from build123d import *

# Parameters (mm, degrees)
EXTRUDE_1_DEPTH     = 14.5
SKETCH_3_W          = 7.5
SKETCH_3_H          = 12.5
CUT_EXTRUDE_1_DEPTH = 14.5
SKETCH_4_W          = 6.236601739
SKETCH_4_H          = 12.5
CUT_EXTRUDE_2_DEPTH = 14.5


with BuildPart() as part:
    # 草图2 → 凸台-拉伸1 (new body)
    with BuildSketch(Plane.XY):
        Polygon((-37.803253111, 45.788749387), (-30.303253111, 45.788749387), (-30.303253111, 46.246753013), (-30.303253111, 51.227331274), (-45.303253111, 51.227331274), (-45.303253111, 45.788749387), align=None)
        with BuildLine():
            Line((-36.53985485, 45.788749387), (-37.803253111, 45.788749387))
            Line((-37.803253111, 45.788749387), (-42.78903224, 11.827146721))
            ThreePointArc((-42.78903224, 11.827146721), (-44.390022844, 0.555474177), (-43.071585345, -10.752730607))
            ThreePointArc((-43.071585345, -10.752730607), (-39.768948275, -19.163531384), (-33.824827731, -25.969147616))
            Line((-33.824827731, -25.969147616), (-33.037880544, -24.9979555))
            ThreePointArc((-33.037880544, -24.9979555), (-38.707558344, -18.503127277), (-41.852353206, -10.475779938))
            ThreePointArc((-41.852353206, -10.475779938), (-43.139798164, 0.565020843), (-41.563632025, 11.568315655))
            Line((-41.563632025, 11.568315655), (-36.53985485, 45.788749387))
        make_face()
    extrude(amount=EXTRUDE_1_DEPTH)

    # 草图3 → 切除-拉伸1 (cut)
    with BuildSketch(Plane.XZ.offset(-45.788749387)):
        with Locations((-41.553253111, 7.25)):
            Rectangle(SKETCH_3_W, SKETCH_3_H)
    extrude(amount=-CUT_EXTRUDE_1_DEPTH, mode=Mode.SUBTRACT)

    # 草图4 → 切除-拉伸2 (cut)
    with BuildSketch(Plane.XZ.offset(-45.788749387)):
        with Locations((-33.421553981, 7.25)):
            Rectangle(SKETCH_4_W, SKETCH_4_H)
    extrude(amount=-CUT_EXTRUDE_2_DEPTH, mode=Mode.SUBTRACT)


solid = part.part
Source: CAD feature listing. Evaluate the final solid. Frame: model axes, mm. A direction names the side the tool comes from. Round coordinates to 2 decimals unless told otherwise and drop trailing zeros. Loops run counter-clockwise (first coordinate to the right, second up) from the corner with the lowest first, then second, coordinate; pieces in that order, holes last. Notation, with made-up numbers: M -31.5,-5 L -7.5,-5 A36 ccw -7.5,30 Z; hole C -14,-10.5 d11. An arc over 180 degrees is marked long. Answer as CSV lines item,"result".
Q1. Cut plane B-B (z = 2). Return the cut outline in (x, y), plus the area to 3 significant figures.
Verdict:
outline,"M -43.07,-10.75 A26.42 ccw -33.82,-25.97 L -33.04,-25 A25.17 cw -41.85,-10.48 A43.14 cw -41.56,11.57 L -36.54,45.79 L -36.54,51.23 L -37.8,51.23 L -37.8,45.79 L -42.79,11.83 A44.39 ccw Z"
area,"100 mm^2"
Q2. Contact query for flat-ended pins moving along their axis: pin 1 (1.6 mm diameter, centred on y = 47.5, z = 8.5, fed in from +X); pin 2 (0.8 mm diameter, centred on x = -32.5, z = 0.5, fed in from -Y); pin 3 (4 mm diameter, centred on x = -41, z = 11.5, fed in from -Y). Output: stop coordinate, or through.
Verdict:
pin 1,"stops at x = -36.54"
pin 2,"stops at y = 45.79"
pin 3,"stops at y = -20.36"
Q3. Line query: line 1 along X through (y, z) = (24, 9.25); line 2 along X through (y, z) = (29.5, 1.5); line 3 along Y through (x, z) = (-34.75, 13). Output: solid intervals per line, ascending.
Verdict:
line 1,"x = -41 to -39.74"
line 2,"x = -40.19 to -38.93"
line 3,"y = -25.18 to -23.48"
Q4. Pull-direction query (Y, two-part tool) for faces 6 (the face through (-33, 48, 1)), 7 (the face through (-39.087, 28.439, 7.148)), 8 (the face through (-39.835, -19.055, 7.148)); classes: +Y half, -Y half, draft (parallel to the pull), parting line (faces both ways), or undercut.
Verdict:
face 6,"draft"
face 7,"undercut"
face 8,"-Y half"
Q5. Cut plane A-A (x = -39). Return the cut outline in (y, z), plus the area to 3 significant figures.
Verdict:
outline,"M -20.36,0 L -18.01,0 L -18.01,14.5 L -20.36,14.5 Z; M 29.03,0 L 37.64,0 L 37.64,14.5 L 29.03,14.5 Z; M 45.79,0 L 51.23,0 L 51.23,1 L 45.79,1 Z; M 45.79,13.5 L 51.23,13.5 L 51.23,14.5 L 45.79,14.5 Z"
area,"170 mm^2"
Q6. Cut plane C-C (y = 37.5). Return the cut outline in (x, z), plus the area to 3 significant figures.
Verdict:
outline,"M -39.02,0 L -37.76,0 L -37.76,14.5 L -39.02,14.5 Z"
area,"18.3 mm^2"
Q7. Cut plane D-D (y = -3). Return the cut outline in (x, z).
Verdict:
outline,"M -44.29,0 L -43.04,0 L -43.04,14.5 L -44.29,14.5 Z"
Q8. Reachability of faces 1 (the face through (-33, 48, 13.5)), 2 (the face through (-40.26, 29.05, 7.15)), 3 (the face through (-42, 48, 13.5)), 4 (the face through (-40, 27, 14.5)), 5 (the face through (-38.64, -18.61, 7.15)) from +Z, -Z, +X, -X, +Y, -Y: full face, straight path, thin tool, end or side. Return the list, or none.
Verdict:
face 1,"+X, +Y"
face 2,"+Z, -Z, -X"
face 3,"-X, +Y"
face 4,"+Z, +X, -X, +Y, -Y"
face 5,"+Z, -Z, +X"
